CAD build for the part. Positions are in the model's coordinates, mm. A direction names the side the tool comes from. Give positions to 0.01 mm unless a question says otherwise; leave off trailing zeros. Write each loop counter-clockwise with the first axis right and the second up, starting at its lowest first coordinate (ties: lowest second). Pieces come first, ordered by that corner, then holes. Notation, with made-up numbers: (-16, 50) - (6, 50) arc R8 cw to (6, 61) - close; hole circle Ø1 at (-27, 69). An arc over 180 degrees is marked (long way). Answer as a JSON object with one key per item and string values.
from build123d import *

# Parameters (mm, degrees)
DODANIE_WYCI_GNI_CIE1_DEPTH = 10
DODANIE_WYCI_GNI_CIE2_DEPTH = 10
SZKIC5_R                    = 1.5
WYTNIJ_WYCI_GNI_CIE1_DEPTH  = 15


with BuildPart() as part:
    # Szkic1 → Dodanie-wyciągnięcie1 (new body)
    with BuildSketch(Plane(origin=(0, 0, 0), x_dir=(1, 0, 0), z_dir=(0, 1, 0))):
        with BuildLine():
            Line((-94.981523654, 75.273037309), (95.018476346, 75.273037309))
            ThreePointArc((95.018476346, 75.273037309), (98.554010252, 73.808571215), (100.018476346, 70.273037309))
            Line((100.018476346, 70.273037309), (100.018476346, -69.726962691))
            ThreePointArc((100.018476346, -69.726962691), (98.554010252, -73.262496597), (95.018476346, -74.726962691))
            Line((95.018476346, -74.726962691), (-94.981523654, -74.726962691))
            ThreePointArc((-94.981523654, -74.726962691), (-98.51705756, -73.262496597), (-99.981523654, -69.726962691))
            Line((-99.981523654, -69.726962691), (-99.981523654, 70.273037309))
            ThreePointArc((-99.981523654, 70.273037309), (-98.51705756, 73.808571215), (-94.981523654, 75.273037309))
        make_face()
    extrude(amount=DODANIE_WYCI_GNI_CIE1_DEPTH)

    # Szkic4 → Dodanie-wyciągnięcie2 (add)
    with BuildSketch(Plane.XZ):
        Polygon((-96, 63.04375976), (-88, 63.04375976), (-88, 71.04375976), (88, 71.04375976), (88, 63.04375976), (96, 63.04375976), (96, -62.95624024), (88, -62.95624024), (88, -70.95624024), (-88, -70.95624024), (-88, -62.95624024), (-96, -62.95624024), align=None)
    extrude(amount=DODANIE_WYCI_GNI_CIE2_DEPTH)

    # Szkic5 → Wytnij-wyciągnięcie1 (cut)
    with BuildSketch(Plane.XZ):
        with Locations(Location((-92, -66.95624024, 0), (0, 0, 270))):
            Circle(SZKIC5_R)
        with Locations(Location((-92, 67.04375976, 0), (0, 0, 270))):
            Circle(SZKIC5_R)
        with Locations(Location((92, 67.04375976, 0), (0, 0, 270))):
            Circle(SZKIC5_R)
        with Locations(Location((92, -66.95624024, 0), (0, 0, 270))):
            Circle(SZKIC5_R)
    extrude(amount=-WYTNIJ_WYCI_GNI_CIE1_DEPTH, mode=Mode.SUBTRACT)


solid = part.part
(1) Probe L1, parallel to Z at x = -92, y = 2.75; L2, parallel to X at y = 5, z = -66; L3, parallel to X at y = -4.5, z = 0.5. List the from-to ranges inside material, lowest first. Write a range as [from, to].
Answer key:
{"L1": "z = [-75.27, -68.46], [-65.46, 65.54], [68.54, 74.73]", "L2": "x = [-99.98, -93.16], [-90.84, 90.84], [93.16, 100.02]", "L3": "x = [-96, 96]"}
(2) Saw through at B-B, the plane x = -61.5. Give the cut face in (y, z).
Answer key:
{"outline": "(-10, -70.96) - (0, -70.96) - (0, -75.27) - (10, -75.27) - (10, 74.73) - (0, 74.73) - (0, 71.04) - (-10, 71.04) - close"}
(3) Saw through at C-C, the plane y = -7.5. Give the cut face in (x, z).
Answer key:
{"outline": "(-96, -62.96) - (-88, -62.96) - (-88, -70.96) - (88, -70.96) - (88, -62.96) - (96, -62.96) - (96, 63.04) - (88, 63.04) - (88, 71.04) - (-88, 71.04) - (-88, 63.04) - (-96, 63.04) - close"}
(4) Flat gauge pins, fed straight in: P1, Ø2.5, axis at y = -3.5, z = 65, coming from the +X side; P2, Ø3, axis at x = -20.5, y = -6.5, coming from the -Z side; P3, Ø9, axis at y = -7, z = -66, coming from the -X side; P4, Ø2.5, axis at x = 92, z = 67.04, coming from the +Y side. Where does each tip first touch, or does it go through?
Answer key:
{"P1": "stops at x = 88", "P2": "stops at z = -70.96", "P3": "stops at x = -96", "P4": "passes through"}
(5) 3-axis set-ups, long thin cutter, end or side, ignore diameter. For faces 1 (the face through (88, -5, 67)), 2 (the face through (-88, -5, 67)), 3 (the face through (-1, -5, 71.044)): which of +Z, -Z, +X, -X, +Y, -Y reach the whole face in a straight line?
Answer key:
{"face 1": "+Z, +X, -Y", "face 2": "+Z, -X, -Y", "face 3": "+Z, +X, -X, -Y"}
(6) Saw through at A-A, the plane z = -9. Give the cut face in (x, y).
Answer key:
{"outline": "(-99.98, 0) - (-96, 0) - (-96, -10) - (96, -10) - (96, 0) - (100.02, 0) - (100.02, 10) - (-99.98, 10) - close"}
